Part model, mm, in its own coordinate system. Face numbers are marked on the shaded views. A direction names the side the tool comes from. Give positions to 0.01 mm unless a question says otherwise; leave off trailing zeros. Order: outer loops, then holes, each group sorted by start corner. A loop starts at its lowest first (then second) coordinate and runs counter-clockwise, first axis right, second up. Notation, with made-up numbers: (-31, 5) - (25, 5) arc R9 cw to (25, 11) - close; hole circle Ø1 at (18, 27). An arc over 180 degrees is marked (long way). One line per item, written item: value.
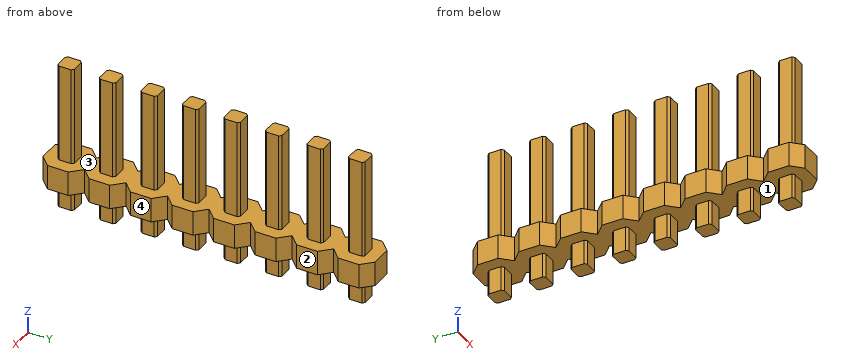
```python
from build123d import *

# Parameters (mm, degrees)
BOSS_EXTRUDE1_DEPTH      = 1.5
BOSS_EXTRUDE2_DEPTH      = 6
BOSS_EXTRUDE2_DEPTH_BACK = 3


with BuildPart() as part:
    # Sketch1 → Boss-Extrude1 (new body)
    with BuildSketch(Plane.XY):
        Polygon((-0.635, 10.16), (0.635, 10.16), (1.27, 9.525), (1.27, 8.255), (0.635, 7.62), (1.27, 6.985), (1.27, 5.715), (0.635, 5.08), (1.27, 4.445), (1.27, 3.175), (0.635, 2.54), (1.27, 1.905), (1.27, 0.635), (0.635, 0), (1.27, -0.635), (1.27, -1.905), (0.635, -2.54), (1.27, -3.175), (1.27, -4.445), (0.635, -5.08), (1.27, -5.715), (1.27, -6.985), (0.635, -7.62), (1.27, -8.255), (1.27, -9.525), (0.635, -10.16), (-0.635, -10.16), (-1.27, -9.525), (-1.27, -8.255), (-0.635, -7.62), (-1.27, -6.985), (-1.27, -5.715), (-0.635, -5.08), (-1.27, -4.445), (-1.27, -3.175), (-0.635, -2.54), (-1.27, -1.905), (-1.27, -0.635), (-0.635, 0), (-1.27, 0.635), (-1.27, 1.905), (-0.635, 2.54), (-1.27, 3.175), (-1.27, 4.445), (-0.635, 5.08), (-1.27, 5.715), (-1.27, 6.985), (-0.635, 7.62), (-1.27, 8.255), (-1.27, 9.525), align=None)
    extrude(amount=BOSS_EXTRUDE1_DEPTH)

    # Sketch2 → Boss-Extrude2 (add, two sides: drawn at the far end of the back side and taken through both)
    with BuildSketch(Plane.XY.offset(1.5).offset(-BOSS_EXTRUDE2_DEPTH_BACK)):
        Polygon((0.375, 9.39), (0.5, 9.265), (0.5, 8.515), (0.375, 8.39), (-0.375, 8.39), (-0.5, 8.515), (-0.5, 9.265), (-0.375, 9.39), align=None)
        Polygon((0.375, 6.85), (0.5, 6.725), (0.5, 5.975), (0.375, 5.85), (-0.375, 5.85), (-0.5, 5.975), (-0.5, 6.725), (-0.375, 6.85), align=None)
        Polygon((0.375, 4.31), (0.5, 4.185), (0.5, 3.435), (0.375, 3.31), (-0.375, 3.31), (-0.5, 3.435), (-0.5, 4.185), (-0.375, 4.31), align=None)
        Polygon((0.375, 1.77), (0.5, 1.645), (0.5, 0.895), (0.375, 0.77), (-0.375, 0.77), (-0.5, 0.895), (-0.5, 1.645), (-0.375, 1.77), align=None)
        Polygon((0.375, -0.77), (0.5, -0.895), (0.5, -1.645), (0.375, -1.77), (-0.375, -1.77), (-0.5, -1.645), (-0.5, -0.895), (-0.375, -0.77), align=None)
        Polygon((0.375, -3.31), (0.5, -3.435), (0.5, -4.185), (0.375, -4.31), (-0.375, -4.31), (-0.5, -4.185), (-0.5, -3.435), (-0.375, -3.31), align=None)
        Polygon((0.375, -5.85), (0.5, -5.975), (0.5, -6.725), (0.375, -6.85), (-0.375, -6.85), (-0.5, -6.725), (-0.5, -5.975), (-0.375, -5.85), align=None)
        Polygon((0.375, -8.39), (0.5, -8.515), (0.5, -9.265), (0.375, -9.39), (-0.375, -9.39), (-0.5, -9.265), (-0.5, -8.515), (-0.375, -8.39), align=None)
    extrude(amount=BOSS_EXTRUDE2_DEPTH + BOSS_EXTRUDE2_DEPTH_BACK)


solid = part.part
```
1) Slice it at A-A on y = -6.5. Write the cut outline in (x, z).
Answer:
outline: (-1.27, 0) - (-0.5, 0) - (-0.5, -1.5) - (0.5, -1.5) - (0.5, 0) - (1.27, 0) - (1.27, 1.5) - (0.5, 1.5) - (0.5, 7.5) - (-0.5, 7.5) - (-0.5, 1.5) - (-1.27, 1.5) - close
2) Wall check: line 1 along Z through (x, y) = (-0.65, -7); line 2 along X through (y, z) = (-7.75, 1.25) (3 decimals); line 3 along X through (y, z) = (-6.75, 5.25) (3 decimals). Give the ranges that are in metal, low to high. Write a range as [from, to].
Answer:
line 1: z = [0, 1.5]
line 2: x = [-0.765, 0.765]
line 3: x = [-0.475, 0.475]
3) Slice it at B-B on x = 1. Count the separate pieces of the cut face and the enclosed holes in it, then the cut area to 3 significant figures.
Answer:
separate pieces: 8
enclosed holes: 0
area: 21.7 mm2
4) Which spindle directions (+Z, -Z, +X, -X, +Y, -Y) get a long thin tool onto all of the face, cutting with end or side? Do the marked faces 3 and 4. Say none if no direction does.
Answer:
face 3: +Z
face 4: +Z, -Z, +X, +Y, -Y
5) Drop flat-ended pins along their axis: P1, Ø0.8, axis at x = 0, z = 3.5, coming from the +Y side; P2, Ø5, axis at y = -5.5, z = 5.5, coming from the -X side; P3, Ø0.6, axis at x = 0, z = 6, coming from the -Y side. Give the stop position or say it passes through.
Answer:
P1: stops at y = 9.39
P2: stops at x = -0.5
P3: stops at y = -9.39
6) Slice it at D-D on y = 2.75. Write the cut outline in (x, z) (3 decimals).
Answer:
outline: (-0.845, 0) - (0.845, 0) - (0.845, 1.5) - (-0.845, 1.5) - close
7) Two-plate mould, pull along Y, no slides. Class the marked faces 1 and 2: pulls with the +Y half, pulls with the -Y half, needs draft (parallel to the pull), parting line crosses it, or undercut.
Answer:
face 1: undercut
face 2: needs draft
